Check sheet for the modelled part. Datum: model origin and axes. Units: mm. A direction names the side the tool comes from. Coordinates: 2 decimals unless noted, no trailing zeros. Loops run counter-clockwise (first coordinate to the right, second up) from the corner with the lowest first, then second, coordinate; pieces in that order, holes last. Notation, with made-up numbers: M 72,26 L 85,26 A17 ccw 85,48 Z; hole C -30.75,-13.5 d5. An arc over 180 degrees is marked long. Answer in a Markdown table with one row per item. Add a question column.
Autodesk Inventor part; units mm, degrees
ref_plane "YZ Plane" through (0, 0, 0) normal (1, 0, 0) x (0, 1, 0)
ref_plane "XZ Plane" through (0, 0, 0) normal (0, 1, 0) x (-1, 0, 0)
ref_plane "XY Plane" through (0, 0, 0) normal (0, 0, 1) x (1, 0, 0)
sketch "Sketch1" plane through (0, 0, 0) normal (0, 0, 1) x (1, 0, 0)
  line L0 (0, 0) -> (25, 0)
  line L1 (25, 0) -> (25, 55.5)
  line L2 (25, 55.5) -> (0, 55.5)
  line L3 (0, 55.5) -> (0, 0)
  dimension "d0" = 25
  dimension "d1" = 55.5
extrude "Extrusion1" add sketch "Sketch1" along normal blind 3
sketch "Sketch2" plane through (0, 0, 3) normal (0, 0, 1) x (1, 0, 0)
  line L0 (0, 55.5) -> (0, 0)
  line L1 (25, 55.5) -> (0, 55.5)
  line L2 (0, 0) -> (3, 0)
  line L3 (3, 0) -> (3, 55.5)
  line L4 (3, 55.5) -> (0, 55.5)
  line L5 (0, 55.5) -> (0, 0)
  dimension "d4" = 3
extrude "Extrusion2" cut sketch "Sketch2" against normal through all
sketch "Sketch3" plane through (0, 0, 3) normal (0, 0, 1) x (1, 0, 0)
  point P0 (0, 0)
sketch "Sketch4" plane through (0, 0, 3) normal (0, 0, 1) x (1, 0, 0)
  line L0 (25, 55.5) -> (3, 55.5)
  line L1 (3, 55.5) -> (18.5, 55.5)
  line L2 (18.5, 55.5) -> (18.5, 22.5)
  line L3 (18.5, 22.5) -> (3, 22.5)
  line L4 (3, 22.5) -> (3, 55.5)
  point P0 (0, 0)
  dimension "d7" = 15.5
  dimension "d8" = 33
sketch "Sketch5" plane through (0, 0, 3) normal (0, 0, 1) x (1, 0, 0)
  line L0 (3, 0) -> (25, 0)
  line L1 (8, 0) -> (18, 0)
  line L2 (18, 0) -> (18, 3)
  line L3 (18, 3) -> (8, 3)
  line L4 (8, 3) -> (8, 0)
  line L5 (3, 55.5) -> (3, 0)
  line L6 (3, 0) -> (8, 0)
  line L7 (8, 0) -> (8, 3)
  line L8 (8, 3) -> (3, 3)
  line L9 (3, 3) -> (3, 0)
  line L10 (18, 0) -> (25, 0)
  line L11 (25, 0) -> (25, 3)
  line L12 (25, 3) -> (18, 3)
  line L13 (18, 3) -> (18, 0)
  point P0 (0, 0)
  point P1 (3, 22.5)
  dimension "d11" = 10
  dimension "d12" = 3
  dimension "d13" = 5
extrude "Extrusion4" cut sketch "Sketch5" against normal through all contours L5 L8 L4 L0 | L2 L12 L11 L0
sketch "Sketch6" plane through (0, 0, 3) normal (0, 0, 1) x (1, 0, 0)
  line L0 (25, 55.5) -> (3, 55.5)
  line L1 (3, 55.5) -> (18.5, 55.5)
  line L2 (18.5, 55.5) -> (18.5, 52.5)
  line L3 (18.5, 52.5) -> (3, 52.5)
  line L4 (3, 52.5) -> (3, 55.5)
  line L5 (18.5, 55.5) -> (18.5, 22.5)
  point P0 (0, 0)
  dimension "d16" = 3
extrude "Extrusion5" cut sketch "Sketch6" against normal through all
sketch "Sketch7" plane through (0, 0, 3) normal (0, 0, 1) x (1, 0, 0)
  line L0 (8, 0) -> (8, 3)
  line L1 (25, 3) -> (18, 3)
  line L2 (8, 0) -> (18, 0)
  line L3 (18, 0) -> (18, 3)
  line L4 (18, 3) -> (8, 3)
  line L5 (8, 3) -> (8, 0)
  point P0 (0, 0)
extrude "Extrusion6" cut sketch "Sketch7" against normal through all
sketch "Sketch8" plane through (0, 0, 3) normal (0, 0, 1) x (1, 0, 0)
  line L0 (3, 3) -> (3, 52.5)
  line L1 (3, 7.5) -> (0, 7.5)
  line L2 (0, 7.5) -> (0, 17.5)
  line L3 (0, 17.5) -> (3, 17.5)
  line L4 (3, 17.5) -> (3, 7.5)
  line L5 (3, 3) -> (25, 3)
  point P0 (0, 0)
  dimension "d21" = 3
  dimension "d22" = 10
  dimension "d23" = 4.5
extrude "Extrusion7" add sketch "Sketch8" against normal blind 3
properties part number "hollow_mount"
Q1. Cross-section at C-C (y = 38). Record the cut outline in (x, z).
Q2. Thickness scan on L1, parallel to X at y = 35, z = 0.3; L2, parallel to Y at x = 14.5, z = 0.7; L3, parallel to Y at x = 1.75, z = 0.1. Record the ranges inside material, lowest first.
Q3. Access from +Z, -Z, +X, -X, +Y, -Y to the whole of each face (thin tool, end or side, straight path). Record for faces 1 (the face through (2, 7.5, 2)), 2 (the face through (22, 55.5, 1)), 3 (the face through (1, 17.5, 2)).
Q4. Go/stop test with flat-tipped pins: pin 1 (1.5 mm diameter, centred on x = 1.5, z = 1.5, fed in from -Y); pin 2 (0.9 mm diameter, centred on y = 54.5, z = 2, fed in from -X); pin 3 (1.5 mm diameter, centred on y = 5.5, z = 1.5, fed in from -X). Record where each tip stops, or that it passes through.
Q5. Cross-section at B-B (x = 5.5). Record the cut outline in (y, z), plus the area to 4 significant figures.
Q6. Cross-section at A-A (z = 1.6). Record the cut outline in (x, y).
Answer key:
| question | item | result |
|---|---|---|
| 1 | outline | M 3,0 L 25,0 L 25,3 L 3,3 Z |
| 2 | L1 | 3 to 25 |
| 2 | L2 | 3 to 52.5 |
| 2 | L3 | 7.5 to 17.5 |
| 3 | face 1 | +Z, -Z, -X, -Y |
| 3 | face 2 | +Z, -Z, +X, -X, +Y |
| 3 | face 3 | +Z, -Z, -X, +Y |
| 4 | pin 1 | y = 7.5 |
| 4 | pin 2 | x = 18.5 |
| 4 | pin 3 | x = 3 |
| 5 | outline | M 3,0 L 52.5,0 L 52.5,3 L 3,3 Z |
| 5 | area | 148.5 mm^2 |
| 6 | outline | M 0,7.5 L 3,7.5 L 3,3 L 25,3 L 25,55.5 L 18.5,55.5 L 18.5,52.5 L 3,52.5 L 3,17.5 L 0,17.5 Z |
